Answer from the drawing. Dimensions are ordinates in mm from the lowest x, y and z of the part. Coordinates: 2 decimals unless noted, no trailing zeros. Loops run counter-clockwise (first coordinate to the right, second up) from the corner with the lowest first, then second, coordinate; pieces in that order, holes last. Notation, with made-up numbers: (5, -22.75) -> (59, -22.75) arc R22 cw to (59, 11.25) -> close; hole circle Ø5 at (12, -33.75). An arc over 180 degrees is marked (long way). Use a Markdown table: item, result.
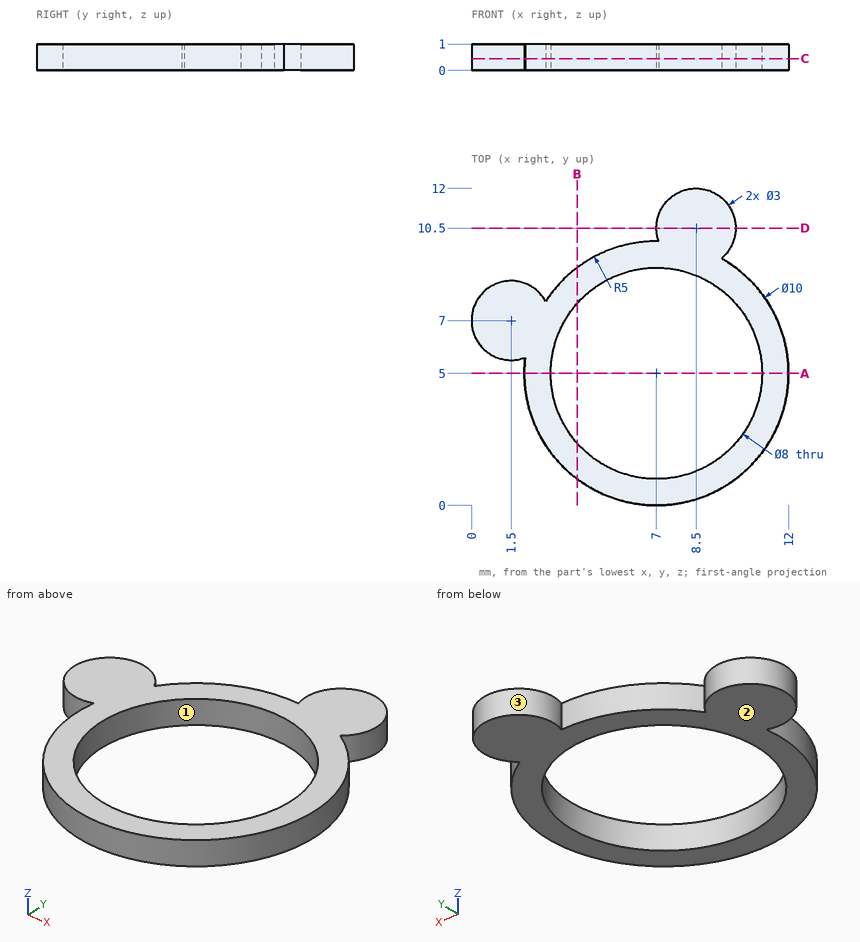
Q1. Section D-D on y = 10.5 is taken. Determine the outline of the cut face in (x, z).
Solved:
| item | result |
|---|---|
| outline | (7, 0) -> (10, 0) -> (10, 1) -> (7, 1) -> close |
Q2. Section B-B on x = 4 is taken. Determine the outline of the cut face in (y, z), and give its area (3 significant figures).
Solved:
| item | result |
|---|---|
| outline | (1, 0) -> (2.35, 0) -> (2.35, 1) -> (1, 1) -> close; (7.65, 0) -> (9, 0) -> (9, 1) -> (7.65, 1) -> close |
| area | 2.71 mm² |
Q3. Determine the mould class of the marked faces 1, 2 and 3 for opening direction Y: pulls with the +Y half, pulls with the -Y half, needs draft (parallel to the pull), parting line crosses it, or undercut.
Solved:
| item | result |
|---|---|
| face 1 | undercut |
| face 2 | needs draft |
| face 3 | undercut |
Q4. Section C-C on z = 0.45 is taken. Determine the outline of the cut face in (x, y).
Solved:
| item | result |
|---|---|
| outline | (2.04, 5.6) arc R5 ccw (long way) to (9.46, 9.35) arc R1.5 ccw (long way) to (7.09, 10) arc R5 ccw to (2.81, 7.73) arc R1.5 ccw (long way) to start; hole circle Ø8 at (7, 5) |
Q5. Consider line 1 (Y direction, x = 7.5, z = 0.8); line 2 (X direction, y = 1.75, z = 0.55); line 3 (X direction, y = 3, z = 0.45). Determine where each line is inside the solid, lowest interval first. Write a range as [from, to].
Solved:
| item | result |
|---|---|
| line 1 | [0.03, 1.03], [8.97, 11.62] |
| line 2 | [3.2, 4.67], [9.33, 10.8] |
| line 3 | [2.42, 3.54], [10.46, 11.58] |
Q6. Section A-A on y = 5 is taken. Determine the outline of the cut face in (x, z).
Solved:
| item | result |
|---|---|
| outline | (2, 0) -> (3, 0) -> (3, 1) -> (2, 1) -> close; (11, 0) -> (12, 0) -> (12, 1) -> (11, 1) -> close |
